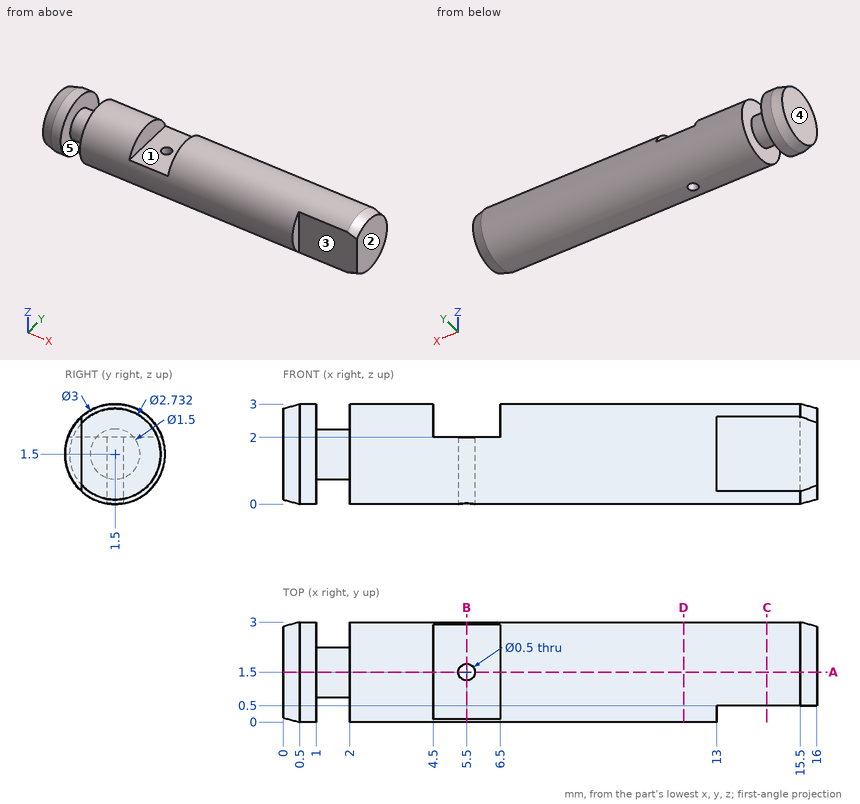
Print and shaded views of the part. All mm, measured from the part's lowest x, y and z. A direction names the side the tool comes from. Give positions to 0.01 mm unless a question says otherwise; leave off trailing zeros. Order: outer loops, then holes, each group sorted by start corner. A loop starts at its lowest first (then second) coordinate and runs counter-clockwise, first axis right, second up. Notation, with made-up numbers: (22, 83.5) - (63, 83.5) arc R23 ccw to (63, 104.5) - close; hole circle Ø3 at (25.25, -21). An arc over 180 degrees is marked (long way). One line per item, written item: value.
Item 1: Wall check: line 1 (X direction, y = 1.5, z = 0.4); line 2 (X direction, y = 1.6, z = 2.3); line 3 (X direction, y = 2.4, z = 0.6). Give the ranges that are in metal, low to high.
Response values:
line 1: 0 to 1, 2 to 5.25, 5.75 to 16
line 2: 0 to 1, 2 to 4.5, 6.5 to 16
line 3: 0 to 1, 2 to 16
Item 2: Slice it at A-A (y = 1.5). List the corners of the cut face in (x, z).
Response values:
outline: (0, 0.13) - (0.5, 0) - (1, 0) - (1, 0.75) - (2, 0.75) - (2, 0) - (5.25, 0) - (5.25, 2) - (4.5, 2) - (4.5, 3) - (2, 3) - (2, 2.25) - (1, 2.25) - (1, 3) - (0.5, 3) - (0, 2.87) - close; (5.75, 0) - (15.5, 0) - (16, 0.13) - (16, 2.87) - (15.5, 3) - (6.5, 3) - (6.5, 2) - (5.75, 2) - close
Item 3: Two-plate mould, pull along X, no slides. Class the marked faces 1, 2 and 3: released by +X, released by -X, zero draft, split by the parting line, or undercut.
Response values:
face 1: undercut
face 2: released by +X
face 3: zero draft
Item 4: Slice it at C-C (x = 14.5). List the corners of the cut face in (y, z).
Response values:
outline: (0.5, 0.38) arc R1.5 ccw (long way) to (0.5, 2.62) - close
Item 5: Slice it at D-D (x = 12). List the corners of the cut face in (y, z).
Response values:
outline: circle Ø3 at (1.5, 1.5)
Item 6: Pin check, flat tip, straight feed: pin 1 Ø1.1 at (x, z) = (15, 1) entering from -Y. Stop position of the tip, or through.
Response values:
pin 1: y = 0.5
Item 7: Tool access for the marked faces 4 and 5: list every direction of +Z, -Z, +X, -X, +Y, -Y with a clear straight run to the whole face (end or side of a thin tool).
Response values:
face 4: +Z, -Z, -X, +Y, -Y
face 5: none
Item 8: Slice it at B-B (x = 5.5). List the corners of the cut face in (y, z), then the cut area to 3 significant figures.
Response values:
outline: (0.09, 2) arc R1.5 ccw to (1.25, 0.02) - (1.25, 2) - close; (1.75, 0.02) arc R1.5 ccw to (2.91, 2) - (1.75, 2) - close
area: 4.01 mm2
